Design review of the part built by this model. Coordinates are the model's own, in mm. Face numbers are marked on the shaded views. A direction names the side the tool comes from. Round coordinates to 2 decimals unless told otherwise and drop trailing zeros. Write each loop counter-clockwise with the first axis right and the second up, starting at its lowest first coordinate (ties: lowest second). Pieces come first, ordered by that corner, then holes. Notation, with made-up numbers: (28, 71) - (73, 71) arc R22 cw to (73, 103) - close; hole circle Ø2 at (79, 39). An arc over 180 degrees is marked (long way). Use one line per item in the form item = value.
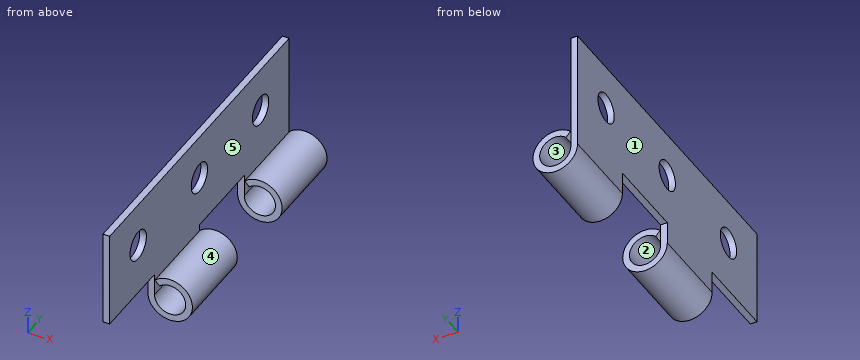
```python
from build123d import *

# Parameters (mm, degrees)
SKETCH1_W           = 13
SKETCH1_H           = 44
BOSS_EXTRUDE1_DEPTH = 0.9
BOSS_EXTRUDE2_DEPTH = 44
SKETCH3_R           = 2
SKETCH3_W           = 6
SKETCH3_H           = 11
CUT_EXTRUDE1_DEPTH  = 127


with BuildPart() as part:
    # Sketch1 → Boss-Extrude1 (new body)
    with BuildSketch(Plane(origin=(0, 0, 0), x_dir=(0, 0, -1), z_dir=(1, 0, 0))):
        with Locations((6.5, 22)):
            Rectangle(SKETCH1_W, SKETCH1_H)
    extrude(amount=BOSS_EXTRUDE1_DEPTH)

    # Sketch2 → Boss-Extrude2 (add)
    with BuildSketch(Plane.XZ):
        with BuildLine():
            Line((0, -16), (0, -13))
            Line((0, -13), (0.9, -13))
            Line((0.9, -13), (0.9, -16))
            ThreePointArc((0.9, -16), (4.925639318, -16.837802611), (1.568488776, -14.46351843))
            Line((1.568488776, -14.46351843), (0.954983966, -13.805026328))
            ThreePointArc((0.954983966, -13.805026328), (5.750913312, -17.196860873), (0, -16))
        make_face()
    extrude(amount=-BOSS_EXTRUDE2_DEPTH)

    # Sketch3 → Cut-Extrude1 (cut)
    with BuildSketch(Plane.ZY):
        with Locations((-6, 7)):
            Circle(SKETCH3_R)
        with Locations((-6, 22)):
            Circle(SKETCH3_R)
        with Locations((-6, 37)):
            Circle(SKETCH3_R)
        with Locations((-16, 5.5)):
            Rectangle(SKETCH3_W, SKETCH3_H)
        with Locations((-16, 27.5)):
            Rectangle(SKETCH3_W, SKETCH3_H)
    extrude(amount=-CUT_EXTRUDE1_DEPTH, mode=Mode.SUBTRACT)


solid = part.part
```
Q1. To check wall thickness, follow line 1 along Y through (x, z) = (0.3, -6); line 2 along X through (y, z) = (35.5, -16); line 3 along Y through (x, z) = (5.2, -17.25). State the ranges of each line that lie inside material, in increasing order. Write a range as from..to.
Calculated:
line_1 = 0..5, 9..20, 24..35, 39..44
line_2 = 0..0.9, 5.1..6
line_3 = 11..22, 33..44
Q2. Draft analysis for pull direction X (two halves, no side actions). For the marked faces 1, 2 and 3, state which applies: released by +X, released by -X, zero draft, split by the parting line, or undercut.
Calculated:
face_1 = released by -X
face_2 = undercut
face_3 = undercut
Q3. For P1, Ø3, axis at x = 2.5, z = -17.5, coming from the +Y side; P2, Ø1, axis at x = 0.5, y = 28.5, coming from the -Z side; P3, Ø6.5, axis at y = 22, z = -6, coming from the +X side, all flat-tipped, find the tip position at first contact; note any pin that passes through.
Calculated:
P1 = 44
P2 = -13
P3 = 0.9
Q4. Machinability: for the marked faces 4 and 5, which of the approach directions +Z, -Z, +X, -X, +Y, -Y give a long, thin tool a straight path to every point of the face, cutting with its end or side? Answer none if there is none.
Calculated:
face_4 = +Y, -Y
face_5 = +Z, +Y, -Y
Q5. We need section C-C on x = 3. Write out the cut boundary in (y, z), then the cut area to 3 significant figures.
Calculated:
outline = (11, -19) - (22, -19) - (22, -18.1) - (11, -18.1) - close; (11, -13.9) - (22, -13.9) - (22, -13) - (11, -13) - close; (33, -19) - (44, -19) - (44, -18.1) - (33, -18.1) - close; (33, -13.9) - (44, -13.9) - (44, -13) - (33, -13) - close
area = 39.6 mm2
Q6. We need section B-B on z = -6. Write out the cut boundary in (x, y), then the cut area to 3 significant figures.
Calculated:
outline = (0, 0) - (0.9, 0) - (0.9, 5) - (0, 5) - close; (0, 9) - (0.9, 9) - (0.9, 20) - (0, 20) - close; (0, 24) - (0.9, 24) - (0.9, 35) - (0, 35) - close; (0, 39) - (0.9, 39) - (0.9, 44) - (0, 44) - close
area = 28.8 mm2
Q7. We need section D-D on x = 5.5. Write out the cut boundary in (y, z), then the cut area to 3 significant figures.
Calculated:
outline = (11, -17.66) - (22, -17.66) - (22, -14.34) - (11, -14.34) - close; (33, -17.66) - (44, -17.66) - (44, -14.34) - (33, -14.34) - close
area = 73.0 mm2
Q8. We need section A-A on y = 37. Write out the cut boundary in (x, z).
Calculated:
outline = (0, -16) arc R3 ccw (long way) to (0.95, -13.81) - (1.57, -14.46) arc R2.1 cw (long way) to (0.9, -16) - (0.9, -8) - (0, -8) - close; (0, -4) - (0.9, -4) - (0.9, 0) - (0, 0) - close
